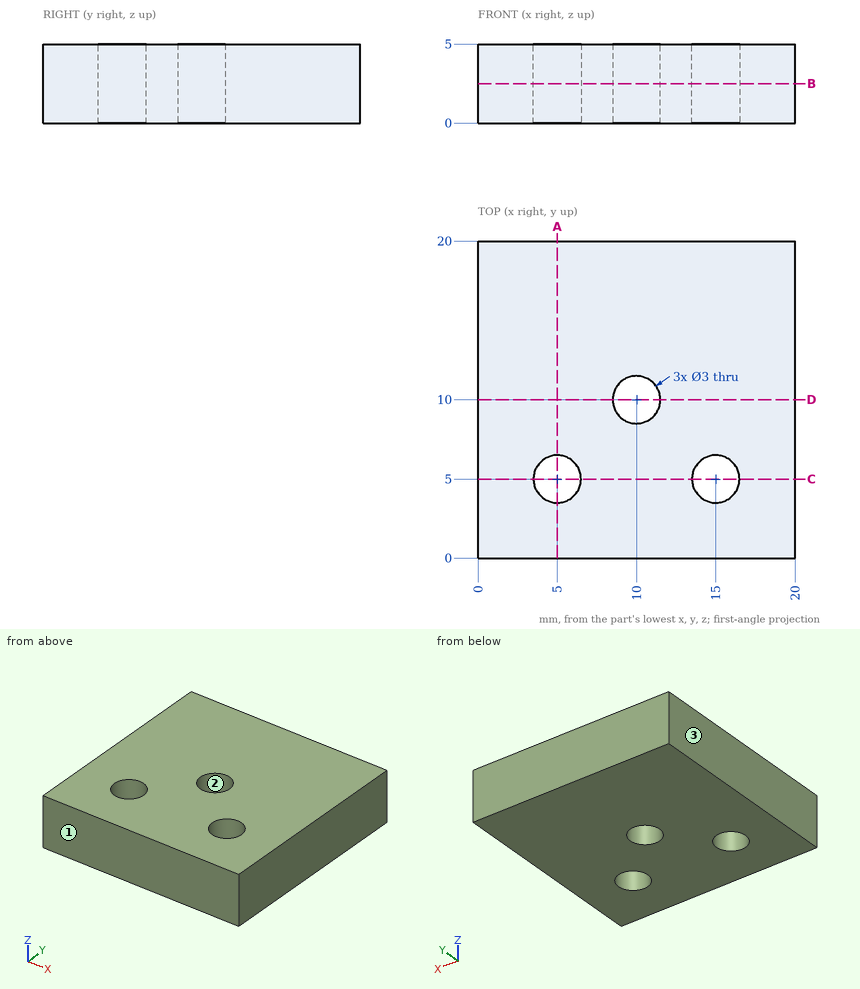
Source: three-view drawing plus pictorial views. Frame: mm from the lowest corner of the part. Give positions to 0.01 mm unless a question says otherwise; leave off trailing zeros. Write each loop counter-clockwise with the first axis right and the second up, starting at its lowest first coordinate (ties: lowest second). Pieces come first, ordered by that corner, then holes.
(1) Mould query, pull axis Y, two halves, no side actions, for the marked faces 1, 2 and 3. Classes: released by +Y, released by -Y, zero draft, split by the parting line, or undercut.
(2) Cut plane B-B, the plane z = 2.5. Return loops of the section in (x, y).
(3) Cut plane C-C, the plane y = 5. Return loops of the section in (x, z).
(4) Cut plane D-D, the plane y = 10. Return loops of the section in (x, z), then the cut area to 3 significant figures.
(5) Ray query, line 1 (Y direction, x = 15, z = 3.65); line 2 (Y direction, x = 4.5, z = 4.1); line 3 (X direction, y = 9.75, z = 4.35). Return the intervals inside material, ascending.
(6) Cut plane A-A, the plane x = 5. Return loops of the section in (y, z).
Values follow:
1. face 1: released by -Y
1. face 2: undercut
1. face 3: zero draft
2. outline: (0, 0) - (20, 0) - (20, 20) - (0, 20) - close; hole circle Ø3 at (5, 5); hole circle Ø3 at (10, 10); hole circle Ø3 at (15, 5)
3. outline: (0, 0) - (3.5, 0) - (3.5, 5) - (0, 5) - close; (6.5, 0) - (13.5, 0) - (13.5, 5) - (6.5, 5) - close; (16.5, 0) - (20, 0) - (20, 5) - (16.5, 5) - close
4. outline: (0, 0) - (8.5, 0) - (8.5, 5) - (0, 5) - close; (11.5, 0) - (20, 0) - (20, 5) - (11.5, 5) - close
4. area: 85.0 mm2
5. line 1: y = 0 to 3.5, 6.5 to 20
5. line 2: y = 0 to 3.59, 6.41 to 20
5. line 3: x = 0 to 8.52, 11.48 to 20
6. outline: (0, 0) - (3.5, 0) - (3.5, 5) - (0, 5) - close; (6.5, 0) - (20, 0) - (20, 5) - (6.5, 5) - close
